```python
from build123d import *

# Parameters (mm, degrees)
SKETCH1_R               = 13.75
SKETCH1_R_2             = 4.1
BOSS_EXTRUDE1_DEPTH     = 2.5
SKETCH2_R               = 6.6
SKETCH2_R_2             = 4.1
BOSS_EXTRUDE2_DEPTH     = 2.5
CUT_EXTRUDE1_DEPTH      = 20.605483927
CUT_EXTRUDE1_DEPTH_BACK = 20.605483927
SKETCH3_R               = 0.75


with BuildPart() as part:
    # Sketch1 → Boss-Extrude1 (new body)
    with BuildSketch(Plane.XY):
        Circle(SKETCH1_R)
        Circle(SKETCH1_R_2, mode=Mode.SUBTRACT)
    extrude(amount=BOSS_EXTRUDE1_DEPTH)

    # Sketch2 → Boss-Extrude2 (add)
    with BuildSketch(Plane.XY.offset(2.5)):
        Circle(SKETCH2_R)
        Circle(SKETCH2_R_2, mode=Mode.SUBTRACT)
    extrude(amount=BOSS_EXTRUDE2_DEPTH)

    # Sketch3 → Cut-Extrude1 (cut, two sides: drawn at the far end of the back side and taken through both)
    with BuildSketch(Plane.XY.offset(2.5).offset(-CUT_EXTRUDE1_DEPTH_BACK)):
        with BuildLine():
            ThreePointArc((0.75, 12), (0, 11.25), (-0.75, 12))
            Line((-0.75, 12), (-0.75, 8.35))
            ThreePointArc((-0.75, 8.35), (0, 9.1), (0.75, 8.35))
            Line((0.75, 8.35), (0.75, 12))
        make_face()
        with BuildLine():
            ThreePointArc((5.285110838, 10.799541816), (4.305188614, 10.393644741), (3.899291539, 11.373566964))
            Line((3.899291539, 11.373566964), (2.502497011, 8.001406671))
            ThreePointArc((2.502497011, 8.001406671), (3.341724402, 8.449983057), (3.94540666, 7.714394096))
            ThreePointArc((3.94540666, 7.714394096), (3.930995621, 7.568076355), (3.88831631, 7.427381522))
            Line((3.88831631, 7.427381522), (5.285110838, 10.799541816))
        make_face()
        with BuildLine():
            ThreePointArc((9.01561146, 7.954951288), (7.954951288, 7.954951288), (7.954951288, 9.01561146))
            Line((7.954951288, 9.01561146), (5.374011537, 6.434671709))
            ThreePointArc((5.374011537, 6.434671709), (6.191354197, 6.597251272), (6.654341623, 5.904341623))
            ThreePointArc((6.654341623, 5.904341623), (6.597251272, 5.617329049), (6.434671709, 5.374011537))
            Line((6.434671709, 5.374011537), (9.01561146, 7.954951288))
        make_face()
        with BuildLine():
            ThreePointArc((11.373566964, 3.899291539), (10.393644741, 4.305188614), (10.799541816, 5.285110838))
            Line((10.799541816, 5.285110838), (7.427381522, 3.88831631))
            ThreePointArc((7.427381522, 3.88831631), (8.131071771, 3.819008869), (8.464394096, 3.19540666))
            ThreePointArc((8.464394096, 3.19540666), (8.337996306, 2.778728985), (8.001406671, 2.502497011))
            Line((8.001406671, 2.502497011), (11.373566964, 3.899291539))
        make_face()
        with BuildLine():
            ThreePointArc((12, -0.75), (11.25, 0), (12, 0.75))
            Line((12, 0.75), (8.35, 0.75))
            ThreePointArc((8.35, 0.75), (8.880330086, 0.530330086), (9.1, 0))
            ThreePointArc((9.1, 0), (8.880330086, -0.530330086), (8.35, -0.75))
            Line((8.35, -0.75), (12, -0.75))
        make_face()
        with BuildLine():
            ThreePointArc((10.799541816, -5.285110838), (10.393644741, -4.305188614), (11.373566964, -3.899291539))
            Line((11.373566964, -3.899291539), (8.001406671, -2.502497011))
            ThreePointArc((8.001406671, -2.502497011), (8.337996306, -2.778728985), (8.464394096, -3.19540666))
            ThreePointArc((8.464394096, -3.19540666), (8.131071771, -3.819008869), (7.427381522, -3.88831631))
            Line((7.427381522, -3.88831631), (10.799541816, -5.285110838))
        make_face()
        with BuildLine():
            ThreePointArc((7.954951288, -9.01561146), (7.954951288, -7.954951288), (9.01561146, -7.954951288))
            Line((9.01561146, -7.954951288), (6.434671709, -5.374011537))
            ThreePointArc((6.434671709, -5.374011537), (6.597251272, -5.617329049), (6.654341623, -5.904341623))
            ThreePointArc((6.654341623, -5.904341623), (6.191354197, -6.597251272), (5.374011537, -6.434671709))
            Line((5.374011537, -6.434671709), (7.954951288, -9.01561146))
        make_face()
        with BuildLine():
            ThreePointArc((3.899291539, -11.373566964), (4.305188614, -10.393644741), (5.285110838, -10.799541816))
            Line((5.285110838, -10.799541816), (3.88831631, -7.427381522))
            ThreePointArc((3.88831631, -7.427381522), (3.930995621, -7.568076355), (3.94540666, -7.714394096))
            ThreePointArc((3.94540666, -7.714394096), (3.341724402, -8.449983057), (2.502497011, -8.001406671))
            Line((2.502497011, -8.001406671), (3.899291539, -11.373566964))
        make_face()
        with BuildLine():
            ThreePointArc((-0.75, -12), (0, -11.25), (0.75, -12))
            Line((0.75, -12), (0.75, -8.35))
            ThreePointArc((0.75, -8.35), (0, -9.1), (-0.75, -8.35))
            Line((-0.75, -8.35), (-0.75, -12))
        make_face()
        with BuildLine():
            ThreePointArc((-3.842201188, -11.08655439), (-3.856612228, -11.232872132), (-3.899291539, -11.373566964))
            Line((-3.899291539, -11.373566964), (-2.502497011, -8.001406671))
            ThreePointArc((-2.502497011, -8.001406671), (-3.482419235, -8.407303746), (-3.88831631, -7.427381522))
            Line((-3.88831631, -7.427381522), (-5.285110838, -10.799541816))
            ThreePointArc((-5.285110838, -10.799541816), (-4.445883447, -10.35096543), (-3.842201188, -11.08655439))
        make_face()
        with BuildLine():
            ThreePointArc((-7.735281374, -8.485281374), (-7.792371725, -8.772293949), (-7.954951288, -9.01561146))
            Line((-7.954951288, -9.01561146), (-5.374011537, -6.434671709))
            ThreePointArc((-5.374011537, -6.434671709), (-6.434671709, -6.434671709), (-6.434671709, -5.374011537))
            Line((-6.434671709, -5.374011537), (-9.01561146, -7.954951288))
            ThreePointArc((-9.01561146, -7.954951288), (-8.1982688, -7.792371725), (-7.735281374, -8.485281374))
        make_face()
        with BuildLine():
            ThreePointArc((-10.33655439, -4.592201188), (-10.462952181, -5.008878863), (-10.799541816, -5.285110838))
            Line((-10.799541816, -5.285110838), (-7.427381522, -3.88831631))
            ThreePointArc((-7.427381522, -3.88831631), (-8.407303746, -3.482419235), (-8.001406671, -2.502497011))
            Line((-8.001406671, -2.502497011), (-11.373566964, -3.899291539))
            ThreePointArc((-11.373566964, -3.899291539), (-10.669876715, -3.968598979), (-10.33655439, -4.592201188))
        make_face()
        with BuildLine():
            ThreePointArc((-11.25, 0), (-11.469669914, -0.530330086), (-12, -0.75))
            Line((-12, -0.75), (-8.35, -0.75))
            ThreePointArc((-8.35, -0.75), (-9.1, 0), (-8.35, 0.75))
            Line((-8.35, 0.75), (-12, 0.75))
            ThreePointArc((-12, 0.75), (-11.469669914, 0.530330086), (-11.25, 0))
        make_face()
        with BuildLine():
            ThreePointArc((-10.33655439, 4.592201188), (-10.669876715, 3.968598979), (-11.373566964, 3.899291539))
            Line((-11.373566964, 3.899291539), (-8.001406671, 2.502497011))
            ThreePointArc((-8.001406671, 2.502497011), (-8.407303746, 3.482419235), (-7.427381522, 3.88831631))
            Line((-7.427381522, 3.88831631), (-10.799541816, 5.285110838))
            ThreePointArc((-10.799541816, 5.285110838), (-10.462952181, 5.008878863), (-10.33655439, 4.592201188))
        make_face()
        with BuildLine():
            ThreePointArc((-7.735281374, 8.485281374), (-8.1982688, 7.792371725), (-9.01561146, 7.954951288))
            Line((-9.01561146, 7.954951288), (-6.434671709, 5.374011537))
            ThreePointArc((-6.434671709, 5.374011537), (-6.434671709, 6.434671709), (-5.374011537, 6.434671709))
            Line((-5.374011537, 6.434671709), (-7.954951288, 9.01561146))
            ThreePointArc((-7.954951288, 9.01561146), (-7.792371725, 8.772293949), (-7.735281374, 8.485281374))
        make_face()
        with BuildLine():
            ThreePointArc((-3.842201188, 11.08655439), (-4.445883447, 10.35096543), (-5.285110838, 10.799541816))
            Line((-5.285110838, 10.799541816), (-3.88831631, 7.427381522))
            ThreePointArc((-3.88831631, 7.427381522), (-3.482419235, 8.407303746), (-2.502497011, 8.001406671))
            Line((-2.502497011, 8.001406671), (-3.899291539, 11.373566964))
            ThreePointArc((-3.899291539, 11.373566964), (-3.856612228, 11.232872132), (-3.842201188, 11.08655439))
        make_face()
        with Locations((0, 12)):
            Circle(SKETCH3_R)
        with Locations((4.592201188, 11.08655439)):
            Circle(SKETCH3_R)
        with Locations((8.485281374, 8.485281374)):
            Circle(SKETCH3_R)
        with Locations((11.08655439, 4.592201188)):
            Circle(SKETCH3_R)
        with Locations((7.714394096, 3.19540666)):
            Circle(SKETCH3_R)
        with Locations((5.904341623, 5.904341623)):
            Circle(SKETCH3_R)
        with Locations((3.19540666, 7.714394096)):
            Circle(SKETCH3_R)
        with Locations((0, 8.35)):
            Circle(SKETCH3_R)
        with Locations((-4.592201188, 11.08655439)):
            Circle(SKETCH3_R)
        with Locations((-8.485281374, 8.485281374)):
            Circle(SKETCH3_R)
        with Locations((-11.08655439, 4.592201188)):
            Circle(SKETCH3_R)
        with Locations((-7.714394096, 3.19540666)):
            Circle(SKETCH3_R)
        with Locations((-5.904341623, 5.904341623)):
            Circle(SKETCH3_R)
        with Locations((-3.19540666, 7.714394096)):
            Circle(SKETCH3_R)
        with Locations((-12, 0)):
            Circle(SKETCH3_R)
        with Locations((-11.08655439, -4.592201188)):
            Circle(SKETCH3_R)
        with Locations((-8.485281374, -8.485281374)):
            Circle(SKETCH3_R)
        with Locations((-4.592201188, -11.08655439)):
            Circle(SKETCH3_R)
        with Locations((-8.35, 0)):
            Circle(SKETCH3_R)
        with Locations((-7.714394096, -3.19540666)):
            Circle(SKETCH3_R)
        with Locations((-5.904341623, -5.904341623)):
            Circle(SKETCH3_R)
        with Locations((-3.19540666, -7.714394096)):
            Circle(SKETCH3_R)
        with Locations((3.19540666, -7.714394096)):
            Circle(SKETCH3_R)
        with Locations((5.904341623, -5.904341623)):
            Circle(SKETCH3_R)
        with Locations((7.714394096, -3.19540666)):
            Circle(SKETCH3_R)
        with Locations((8.35, 0)):
            Circle(SKETCH3_R)
        with Locations((12, 0)):
            Circle(SKETCH3_R)
        with Locations((11.08655439, -4.592201188)):
            Circle(SKETCH3_R)
        with Locations((8.485281374, -8.485281374)):
            Circle(SKETCH3_R)
        with Locations((4.592201188, -11.08655439)):
            Circle(SKETCH3_R)
        with Locations((0, -12)):
            Circle(SKETCH3_R)
        with Locations((0, -8.35)):
            Circle(SKETCH3_R)
    extrude(amount=CUT_EXTRUDE1_DEPTH + CUT_EXTRUDE1_DEPTH_BACK, mode=Mode.SUBTRACT)


solid = part.part
```
Geometry: final body of the model. Coordinates: model frame, mm. A direction names the side the tool comes from. Give positions to 0.01 mm unless a question says otherwise; leave off trailing zeros. Order: outer loops, then holes, each group sorted by start corner. A loop starts at its lowest first (then second) coordinate and runs counter-clockwise, first axis right, second up. Notation, with made-up numbers: M 89,88 L 132,88 A25 cw 132,100 Z; hole C -3,70.5 d5. An arc over 180 degrees is marked long. Answer as CSV lines item,"result". Start each with the question number.
1) Cut plane B-B (x = 0). Output: boundary loops of the cut face in (y, z), then the cut area to 3 significant figures.
2) Mould query, pull axis Y, two halves, no side actions, for faces 3 (the flat face through (5.92, 3.25, 2.5)), 4 (the flat face through (-4.577, -9.09, 1.233)). Classes: +Y half, -Y half, draft (parallel to the pull), parting line (faces both ways), or undercut.
3) Cut plane C-C (z = 4.2). Output: boundary loops of the cut face in (x, y), then the cut area to 3 significant figures.
4) Line query: line 1 (Y direction, x = 0, z = 2.2); line 2 (Y direction, x = 0, z = 3.5); line 3 (Y direction, x = -11, z = 1.6). Output: solid intervals per line, ascending. Write a range as from..to.
5) First-contact query: P1, Ø2, axis at y = 11, z = 2, coming from the -X side; P2, Ø1.2, axis at x = -9.5, z = 2, coming from the +Y side; P3, Ø1, axis at y = -4, z = 1, coming from the -X side. Flat tips, straight axial feed; report the tip coordinate or a pass-through.
6) Cut plane D-D (x = -4.75). Output: boundary loops of the cut face in (y, z).
7) Cut plane A-A (y = -4.5). Output: boundary loops of the cut face in (x, z).
8) Set-up query: faces 1 (the flat face through (2.9, 3.2, 0)), 2 (the cylindrical face through (-7.6, 0, 1.2)). Return all of +Z, -Z, +X, -X, +Y, -Y with unobstructed straight access to the full face (end or side cutting, diameter ignored); none if empty.
Findings below:
1,outline,"M -13.75,0 L -12.75,0 L -12.75,2.5 L -13.75,2.5 Z; M -7.6,0 L -4.1,0 L -4.1,5 L -6.6,5 L -6.6,2.5 L -7.6,2.5 Z; M 4.1,0 L 7.6,0 L 7.6,2.5 L 6.6,2.5 L 6.6,5 L 4.1,5 Z; M 12.75,0 L 13.75,0 L 13.75,2.5 L 12.75,2.5 Z"
1,area,"35.0 mm²"
2,face 3,"draft"
2,face 4,"undercut"
3,outline,"C 0,0 d13.2; hole C 0,0 d8.2"
3,area,"84.0 mm²"
4,line 1,"y = -13.75..-12.75, -7.6..-4.1, 4.1..7.6, 12.75..13.75"
4,line 2,"y = -6.6..-4.1, 4.1..6.6"
4,line 3,"y = -8.25..-5.34, -3.74..-0.75, 0.75..3.74, 5.34..8.25"
5,P1,"stops at x = -9.44"
5,P2,"stops at y = 10.48"
5,P3,"stops at x = -13.3"
6,outline,"M -12.9,0 L -11.82,0 L -11.82,2.5 L -12.9,2.5 Z; M -9.51,0 L 9.51,0 L 9.51,2.5 L 4.58,2.5 L 4.58,5 L -4.58,5 L -4.58,2.5 L -9.51,2.5 Z; M 11.82,0 L 12.9,0 L 12.9,2.5 L 11.82,2.5 Z"
7,outline,"M -12.99,0 L -11.83,0 L -11.83,2.5 L -12.99,2.5 Z; M -8.9,0 L 8.9,0 L 8.9,2.5 L 4.83,2.5 L 4.83,5 L -4.83,5 L -4.83,2.5 L -8.9,2.5 Z; M 11.83,0 L 12.99,0 L 12.99,2.5 L 11.83,2.5 Z"
8,face 1,"-Z, +X, -X, +Y, -Y"
8,face 2,"+Z, -Z"
